from build123d import *

# Parameters (mm, degrees)
F1_DEPTH = 6.35


with BuildPart() as f1:
    # F0 (on Right) → F1 (new body)
    with BuildSketch(Plane.YZ):
        with BuildLine():
            ThreePointArc((12.7, -6.35), (7.193167, -1.488666), (0, 0))
            Line((0, 0), (0, -31.75))
            Line((0, -31.75), (25.4, -31.75))
            Line((25.4, -31.75), (25.4, -25.4))
            Line((25.4, -25.4), (12.7, -6.35))
        make_face()
    extrude(amount=F1_DEPTH)


solid = f1.part
Part model, mm, in its own coordinate system. Coordinates: 2 decimals unless noted, no trailing zeros. Loops run counter-clockwise (first coordinate to the right, second up) from the corner with the lowest first, then second, coordinate; pieces in that order, holes last. Notation, with made-up numbers: M 28.5,-13 L 83.5,-13 A30 ccw 83.5,16 Z; hole C 4.25,6.5 d2. An arc over 180 degrees is marked long. Use a Markdown table: item, result. Add a question column.
Q1. Cut at C-C (z = -11). Write the cut outline in (x, y), and give its area (3 significant figures).
Q2. Pin check, flat tip, straight feed: P1, Ø5, axis at y = 13, z = -4, coming from the -X side. Stop position of the tip, or through.
Q3. Cut at B-B (y = 16.5). Write the cut outline in (x, z).
Q4. Cut at A-A (x = 4). Write the cut outline in (y, z), and give its area (3 significant figures).
Q5. Probe L1, parallel to Z at x = 2, y = 1.5; L2, parallel to Y at x = 5.5, z = -3; L3, parallel to Z at x = 2.5, y = 9. List the from-to ranges inside material, lowest first.
Worked out:
| question | item | result |
|---|---|---|
| 1 | outline | M 0,0 L 6.35,0 L 6.35,15.8 L 0,15.8 Z |
| 1 | area | 100 mm2 |
| 2 | P1 | stops at x = 0 |
| 3 | outline | M 0,-31.75 L 6.35,-31.75 L 6.35,-12.05 L 0,-12.05 Z |
| 4 | outline | M 0,-31.75 L 25.4,-31.75 L 25.4,-25.4 L 12.7,-6.35 A14.31 ccw 0,0 Z |
| 4 | area | 583 mm2 |
| 5 | L1 | z = -31.75 to 0 |
| 5 | L2 | y = 0 to 9.59 |
| 5 | L3 | z = -31.75 to -2.56 |
